The model under review builds one solid part; all positions refer to its coordinate system, in mm. Face numbers are marked on the shaded views. A direction names the side the tool comes from. Give positions to 0.01 mm unless a question says otherwise; leave off trailing zeros. Loops run counter-clockwise (first coordinate to the right, second up) from the corner with the lowest first, then second, coordinate; pieces in that order, holes last. Notation, with made-up numbers: M -25,-35.5 L 25,-35.5 A17 ccw 25,-5.5 Z; hole C -31.75,23 d6. An arc over 180 degrees is marked long. Put each result on its own line as item: value. Start each with the question number.
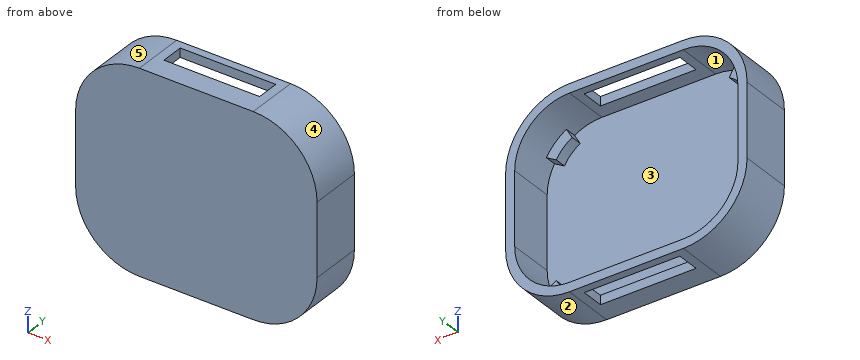
```python
from build123d import *

# Parameters (mm, degrees)
BOSS_EXTRUDE1_DEPTH     = 5.75
CUT_EXTRUDE1_DEPTH      = 50.993124527
CUT_EXTRUDE1_DEPTH_BACK = 50.993124527
SKETCH2_W               = 21
SKETCH2_H               = 5
BOSS_EXTRUDE2_START     = -1.5
BOSS_EXTRUDE2_DEPTH     = 1.5
BOSS_EXTRUDE3_START     = 2.5
BOSS_EXTRUDE3_DEPTH     = 2.5


with BuildPart() as part:
    # Sketch1 → Boss-Extrude1 (new, symmetric)
    with BuildSketch(Plane(origin=(0, 0, 0), x_dir=(1, 0, 0), z_dir=(0, 1, 0))):
        with BuildLine():
            Line((-26.5, 8), (-26.5, -8))
            ThreePointArc((-26.5, -8), (-22.399494937, -17.899494937), (-12.5, -22))
            Line((-12.5, -22), (12.5, -22))
            ThreePointArc((12.5, -22), (22.399494937, -17.899494937), (26.5, -8))
            Line((26.5, -8), (26.5, 8))
            ThreePointArc((26.5, 8), (22.399494937, 17.899494937), (12.5, 22))
            Line((12.5, 22), (-12.5, 22))
            ThreePointArc((-12.5, 22), (-22.399494937, 17.899494937), (-26.5, 8))
        make_face()
        with BuildLine():
            Line((12.5, -20), (-12.5, -20))
            ThreePointArc((-12.5, -20), (-20.985281374, -16.485281374), (-24.5, -8))
            Line((-24.5, -8), (-24.5, 8))
            ThreePointArc((-24.5, 8), (-20.985281374, 16.485281374), (-12.5, 20))
            Line((-12.5, 20), (12.5, 20))
            ThreePointArc((12.5, 20), (20.985281374, 16.485281374), (24.5, 8))
            Line((24.5, 8), (24.5, -8))
            ThreePointArc((24.5, -8), (20.985281374, -16.485281374), (12.5, -20))
        make_face(mode=Mode.SUBTRACT)
    extrude(amount=BOSS_EXTRUDE1_DEPTH, both=True)

    # Sketch2 → Cut-Extrude1 (cut, two sides: drawn at the far end of the back side and taken through both)
    with BuildSketch(Plane.XY.offset(-20).offset(-CUT_EXTRUDE1_DEPTH_BACK)):
        with Locations((0, 1.5)):
            Rectangle(SKETCH2_W, SKETCH2_H)
    extrude(amount=CUT_EXTRUDE1_DEPTH + CUT_EXTRUDE1_DEPTH_BACK, mode=Mode.SUBTRACT)

    # Sketch3 → Boss-Extrude2 (add)
    with BuildSketch(Plane.XZ.offset(5.75).offset(BOSS_EXTRUDE2_START)):
        with BuildLine():
            Line((-12.5, -22), (12.5, -22))
            ThreePointArc((12.5, -22), (22.399494937, -17.899494937), (26.5, -8))
            Line((26.5, -8), (26.5, 8))
            ThreePointArc((26.5, 8), (22.399494937, 17.899494937), (12.5, 22))
            Line((12.5, 22), (-12.5, 22))
            ThreePointArc((-12.5, 22), (-22.399494937, 17.899494937), (-26.5, 8))
            Line((-26.5, 8), (-26.5, -8))
            ThreePointArc((-26.5, -8), (-22.399494937, -17.899494937), (-12.5, -22))
        make_face()
    extrude(amount=BOSS_EXTRUDE2_DEPTH)

    # Sketch6 → Boss-Extrude3 (add)
    with BuildSketch(Plane(origin=(0, -4.25, 0), x_dir=(1, 0, 0), z_dir=(0, 1, 0)).offset(BOSS_EXTRUDE3_START)):
        with BuildLine():
            Line((-22.892304845, 14), (-20.727241336, 12.75))
            ThreePointArc((-20.727241336, 12.75), (-19.217514421, 14.717514421), (-17.25, 16.227241336))
            Line((-17.25, 16.227241336), (-18.5, 18.392304845))
            ThreePointArc((-18.5, 18.392304845), (-20.985281374, 16.485281374), (-22.892304845, 14))
        make_face()
        with BuildLine():
            Line((17.25, 16.227241336), (18.5, 18.392304845))
            ThreePointArc((18.5, 18.392304845), (20.985281374, 16.485281374), (22.892304845, 14))
            Line((22.892304845, 14), (20.727241336, 12.75))
            ThreePointArc((20.727241336, 12.75), (19.217514421, 14.717514421), (17.25, 16.227241336))
        make_face()
        with BuildLine():
            Line((22.892304845, -14), (20.727241336, -12.75))
            ThreePointArc((20.727241336, -12.75), (19.217514421, -14.717514421), (17.25, -16.227241336))
            Line((17.25, -16.227241336), (18.5, -18.392304845))
            ThreePointArc((18.5, -18.392304845), (20.985281374, -16.485281374), (22.892304845, -14))
        make_face()
        with BuildLine():
            Line((-17.25, -16.227241336), (-18.5, -18.392304845))
            ThreePointArc((-18.5, -18.392304845), (-20.985281374, -16.485281374), (-22.892304845, -14))
            Line((-22.892304845, -14), (-20.727241336, -12.75))
            ThreePointArc((-20.727241336, -12.75), (-19.217514421, -14.717514421), (-17.25, -16.227241336))
        make_face()
    extrude(amount=-BOSS_EXTRUDE3_DEPTH)


solid = part.part
```
Item 1: Consider section A-A, the plane y = 1.25. Write out the cut boundary in (x, z).
Item 2: Consider section B-B, the plane x = 0. Write out the cut boundary in (y, z), plus the area to 3 significant figures.
Item 3: Tool access review of the marked faces 1 and 2: name each direction out of +Z, -Z, +X, -X, +Y, -Y from which nothing blocks a thin tool from reaching the whole face with its end or side.
Item 4: Consider section C-C, the plane z = 1. Write out the cut boundary in (x, y).
Item 5: Clearance check with flat-ended pins moving along their axes: pin 1 Ø5 at (x, y) = (-16.5, 1.5) entering from -Z; pin 2 Ø1.6 at (y, z) = (2, -21) entering from +X; pin 3 Ø2 at (y, z) = (1.5, -21.5) entering from -X. State where each tip first meets the part, or that it passes through.
Item 6: To check wall thickness, follow L1, parallel to X at y = -1.25, z = -2.5; L2, parallel to Z at x = -10, y = -1.5; L3, parallel to Y at x = -1, z = -15. State the ranges of each line that lie inside material, in increasing order. Write a range as [from, to].
Item 7: Draft analysis for pull direction X (two halves, no side actions). For the marked faces 3, 4 and 5, state which applies: +X half, -X half, draft (parallel to the pull), parting line (faces both ways), or undercut.
Report:
1. outline: M -26.5,-8 A14 ccw -12.5,-22 L -10.5,-22 L -10.5,-20 L -12.5,-20 A12 cw -24.5,-8 L -24.5,8 A12 cw -12.5,20 L -10.5,20 L -10.5,22 L -12.5,22 A14 ccw -26.5,8 Z; M 10.5,-22 L 12.5,-22 A14 ccw 26.5,-8 L 26.5,8 A14 ccw 12.5,22 L 10.5,22 L 10.5,20 L 12.5,20 A12 cw 24.5,8 L 24.5,-8 A12 cw 12.5,-20 L 10.5,-20 Z
2. outline: M -5.75,-22 L -1,-22 L -1,-20 L -4.25,-20 L -4.25,20 L -1,20 L -1,22 L -5.75,22 Z; M 4,-22 L 5.75,-22 L 5.75,-20 L 4,-20 Z; M 4,20 L 5.75,20 L 5.75,22 L 4,22 Z
2. area: 86.0 mm²
3. face 1: +Y
3. face 2: -Z, +X, +Y, -Y
4. outline: M -26.5,-5.75 L 26.5,-5.75 L 26.5,5.75 L 24.5,5.75 L 24.5,-4.25 L -24.5,-4.25 L -24.5,5.75 L -26.5,5.75 Z
5. pin 1: z = -21.92
5. pin 2: x = 19.37
5. pin 3: x = -18.8
6. L1: [-26.5, -24.5], [24.5, 26.5]
6. L2: [-22, -20], [20, 22]
6. L3: [-5.75, -4.25]
7. face 3: undercut
7. face 4: +X half
7. face 5: -X half
